Source: CAD feature listing. Evaluate the final solid. Frame: model axes, mm. Face numbers are marked on the shaded views. Coordinates: 2 decimals unless noted, no trailing zeros. Order: outer loops, then holes, each group sorted by start corner. A loop starts at its lowest first (then second) coordinate and runs counter-clockwise, first axis right, second up. Notation, with made-up numbers: (-25.5, 65) - (14.5, 65) arc R16 cw to (14.5, 75) - close; hole circle Ø9 at (56.25, 52.5). An arc over 180 degrees is marked (long way). One line per question, with ' | ' between items. Start each with the question number.
(1) Section A-A (x = 0). Return the cut outline in (y, z), then the cut area to 3 significant figures.
(2) Draft query along X for the marked faces 1, 2 and 3. Return one class per face: +X half, -X half, draft (parallel to the pull), parting line (faces both ways), or undercut.
(3) Contact query for flat-ended pins moving along their axis: P1, Ø4, axis at x = 33.04, z = 9.61, coming from the +Y side; P2, Ø12, axis at x = -11.5, y = -10.5, coming from the -Z side; P3, Ø8, axis at y = -13.5, z = 10.5, coming from the +X side. Output: stop coordinate, or through.
(4) Section C-C (x = 33). Return the cut outline in (y, z).
(5) Section B-B (y = 0). Return the cut outline in (x, z), then the cut area to 3 significant figures.
(6) Line query: line 1 along X through (y, z) = (-9, 9.25); line 2 along X through (y, z) = (-18, 8); line 3 along Z through (x, y) = (0, -10). Output: solid intervals per line, ascending.
from build123d import *

# Parameters (mm, degrees)
F0_R     = 2.38125
F1_DEPTH = 12.7
F2_DEPTH = 25.4
F3_DEPTH = 25.4
F4_DEPTH = 25.4


# Not quite as in the source:
# - a feature names something its author has since deleted; it is built from what else it names


with BuildPart() as f1:
    # F0 (on Front) → F1 (new body, symmetric)
    with BuildSketch(Plane.XZ):
        Polygon((-45.6028679988, 0), (46.4721320012, 0), (45.7215224688, 19.5158975394), (-45.6028679988, 19.5158975394), align=None)
        with Locations((33.0442860723, 9.6084093675)):
            Circle(F0_R, mode=Mode.SUBTRACT)
        with Locations((-25.7945582271, 9.7579487697)):
            Circle(F0_R, mode=Mode.SUBTRACT)
        with Locations((0, 10.9073175117)):
            Circle(F0_R, mode=Mode.SUBTRACT)
    extrude(amount=F1_DEPTH, both=True)

    # F0 (on Front) → F2 (join)
    with BuildSketch(Plane.XZ):
        Polygon((-45.6028679988, 0), (46.4721320012, 0), (45.7215224688, 19.5158975394), (-45.6028679988, 19.5158975394), align=None)
        with Locations((33.0442860723, 9.6084093675)):
            Circle(F0_R, mode=Mode.SUBTRACT)
        with Locations((-25.7945582271, 9.7579487697)):
            Circle(F0_R, mode=Mode.SUBTRACT)
        with Locations((0, 10.9073175117)):
            Circle(F0_R, mode=Mode.SUBTRACT)
    extrude(amount=F2_DEPTH)

    # F0 (on Front) → F3 (join)
    with BuildSketch(Plane.XZ):
        Polygon((-45.6028679988, 0), (46.4721320012, 0), (45.7215224688, 19.5158975394), (-45.6028679988, 19.5158975394), align=None)
        with Locations((33.0442860723, 9.6084093675)):
            Circle(F0_R, mode=Mode.SUBTRACT)
        with Locations((-25.7945582271, 9.7579487697)):
            Circle(F0_R, mode=Mode.SUBTRACT)
        with Locations((0, 10.9073175117)):
            Circle(F0_R, mode=Mode.SUBTRACT)
    extrude(amount=F3_DEPTH)

    # F0 (on Front) → F4 (join)
    with BuildSketch(Plane.XZ):
        Polygon((-45.6028679988, 0), (46.4721320012, 0), (45.7215224688, 19.5158975394), (-45.6028679988, 19.5158975394), align=None)
        with Locations((33.0442860723, 9.6084093675)):
            Circle(F0_R, mode=Mode.SUBTRACT)
        with Locations((-25.7945582271, 9.7579487697)):
            Circle(F0_R, mode=Mode.SUBTRACT)
        with Locations((0, 10.9073175117)):
            Circle(F0_R, mode=Mode.SUBTRACT)
    extrude(amount=F4_DEPTH)


solid = f1.part
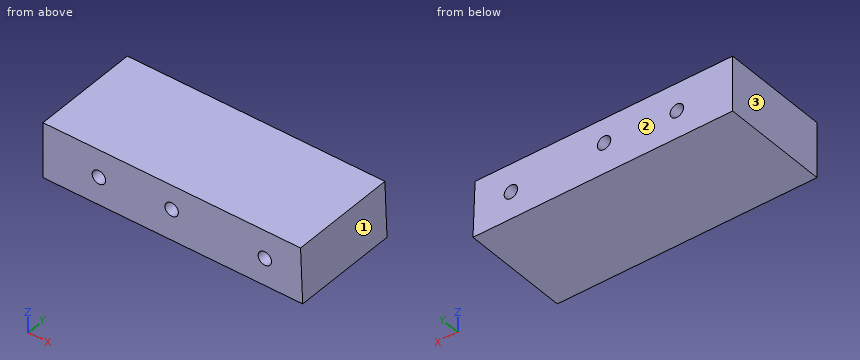
Response values:
1) outline: (-25.4, 0) - (12.7, 0) - (12.7, 8.53) - (-25.4, 8.53) - close; (-25.4, 13.29) - (12.7, 13.29) - (12.7, 19.52) - (-25.4, 19.52) - close | area: 562 mm²
2) face 1: +X half | face 2: draft | face 3: -X half
3) P1: passes through | P2: stops at z = 0 | P3: stops at x = 46.22
4) outline: (-25.4, 0) - (12.7, 0) - (12.7, 7.23) - (-25.4, 7.23) - close; (-25.4, 11.99) - (12.7, 11.99) - (12.7, 19.52) - (-25.4, 19.52) - close
5) outline: (-45.6, 0) - (46.47, 0) - (45.72, 19.52) - (-45.6, 19.52) - close; hole circle Ø4.76 at (-25.79, 9.76); hole circle Ø4.76 at (0, 10.91); hole circle Ø4.76 at (33.04, 9.61) | area: 1,740 mm²
6) line 1: x = -45.6 to -28.12, -23.47 to -1.71, 1.71 to 30.69, 35.4 to 46.12 | line 2: x = -45.6 to -27.4, -24.19 to 31.29, 34.8 to 46.16 | line 3: z = 0 to 8.53, 13.29 to 19.52
